Solid Edge part; units mm, degrees
sketch "Sketch1" plane through (0, 0, 0) normal (1, 0, 0) x (0, 1, 0)
  line L0 (0, -1.6764) -> (0, 1.6764)
  arc A0 (0, 1.6764) -> (5.55625, -1.6764) centre (-0.25374, -5.024398) cw
  line L1 (0, -1.6764) -> (5.55625, -1.6764)
revolve "RevolvedProtrusion1" add sketch "Sketch1" angle 360 about axis through (0, 0, -14.779625) along (0, 0, 1)
sketch "Sketch2" plane through (0, 0, -1.6764) normal (0, 0, -1) x (0, 1, 0)
  circle A0 centre (0, 0) radius 3.175
extrude "Protrusion1" add sketch "Sketch2" along normal blind 31.75
sketch "Sketch3" plane through (0, 0, -33.4264) normal (0, 0, -1) x (1, 0, 0)
  circle A0 centre (0, 0) radius 3.17246
extrude "Cutout1" cut sketch "Sketch3" against normal blind 30.1625 flip side to cut
sketch "Sketch4" plane through (-0.603226, 0.360624, 3.3528) normal (0, 0, 1) x (1, 0, 0)
  line L0 (-0.542454, 1.623751) -> (1.748905, 1.623751)
  line L1 (2.894585, -0.360624) -> (1.748905, 1.623751)
  line L2 (1.748905, -2.344999) -> (2.894585, -0.360624)
  line L3 (-0.542454, -2.344999) -> (1.748905, -2.344999)
  line L4 (-1.688133, -0.360624) -> (-0.542454, -2.344999)
  line L5 (-0.542454, 1.623751) -> (-1.688133, -0.360624)
extrude "ExtrudedCutout_11" cut sketch "Sketch4" against normal blind 5.0292
properties part number "171348"
Could you check a few things on this model? Use its own coordinates, in mm. A direction names the side the tool comes from. Coordinates: 2 decimals unless noted, no trailing zeros. Loops run counter-clockwise (first coordinate to the right, second up) from the corner with the lowest first, then second, coordinate; pieces in that order, holes last.
1. Imagine slicing it at A-A (z = -24). Please give me the cut outline in (x, y).
2. For faces 5 (the face through (2.4, 2.4, -1.676)), 6 (the face through (0, -1.984, 0)), which set-ups out of +Z, -Z, +X, -X, +Y, -Y let a thin tool reach every point of the face, with its end or its side?
3. We'd pull the mould along Y, two halves only. Please class faces 1 (the face through (0, 0, -33.426)), 2 (the face through (1.727, 0.978, -0.169)), 3 (the face through (1.71, -1.01, -0.17)), 4 (the face through (3.1, -0.69, -2.46)): released by +Y, released by -Y, zero draft, split by the parting line, or undercut.
4. I need wall thicknesses on L1, parallel to Y at x = -1.25, z = -0.5; L2, parallel to Z at x = 4.25, y = 0.5; L3, parallel to Y at x = -2, z = -23. Which ranges of each line are inside material? Lowest first, please.
5. For P1, Ø1, axis at x = -0.5, z = -24, coming from the +Y side; P2, Ø2, axis at x = 1.5, z = -19.5, coming from the -Y side; P3, Ø1.8, axis at x = 0.5, z = 0.5, coming from the +Y side, each with a flat end and sliding along its axis, tell me the tip position at first contact or that it passes through.
Computed values:
1. outline: circle Ø6.34 at (0, 0)
2. face 5: -Z
2. face 6: +Z
3. face 1: zero draft
3. face 2: undercut
3. face 3: undercut
3. face 4: split by the parting line
4. L1: y = -4.53 to -1.8, 1.8 to 4.53
4. L2: z = -1.68 to -0.08
4. L3: y = -2.46 to 2.46
5. P1: stops at y = 3.17
5. P2: stops at y = -3.13
5. P3: stops at y = 4.58
